Autodesk Inventor part; units mm, degrees
ref_plane "YZ Plane" through (0, 0, 0) normal (1, 0, 0) x (0, 1, 0)
ref_plane "XZ Plane" through (0, 0, 0) normal (0, 1, 0) x (-1, 0, 0)
ref_plane "XY Plane" through (0, 0, 0) normal (0, 0, 1) x (1, 0, 0)
sketch "Sketch1" plane through (0, 0, 0) normal (0, 1, 0) x (-1, 0, 0)
  line L0 (217.0075, 238.5115) -> (-11.2469, 238.5115)
  line L1 (-36.6469, 213.1115) -> (-36.6469, 88.1828)
  line L2 (-11.5925, 62.7851) -> (215.7472, 62.7851)
  line L3 (241.1469, 88.0591) -> (241.1469, 213.1428)
  arc A0 (217.0075, 238.5115) -> (241.1469, 213.1428) centre (242.4075, 238.5115) ccw
  arc A1 (241.1469, 88.0591) -> (215.7472, 62.7851) centre (241.1469, 62.6591) ccw
  arc A2 (-36.6469, 213.1115) -> (-11.2469, 238.5115) centre (-36.6469, 238.5115) ccw
  arc A3 (-11.5925, 62.7851) -> (-36.6469, 88.1828) centre (-36.9925, 62.7851) ccw
  circle A4 centre (215.7469, 150.6529) radius 9.525
  circle A5 centre (215.7469, 150.6529) radius 6.35
  point P0 (0, 0)
  dimension "d6" = 227.3398
  dimension "d7" = 277.7939
  dimension "d10" = 125.0838
  dimension "d11" = 175.7264
  dimension "d12" = 19.05
  dimension "d13" = 12.7
  dimension "d14" = 87.8586
  dimension "d15" = 25.4
extrude "Extrusion1" add sketch "Sketch1" along normal blind 25.4 contours A0 L3 A1 L2 A3 L1 A2 L0 | A4 | A5
extrude "Extrusion2" cut sketch "Sketch1" along normal blind 5.08 contours A5
sketch "Sketch2" plane through (0, 0, 0) normal (0, -1, 0) x (1, 0, 0)
  point P0 (0, 0)
sketch "Sketch3" plane through (0, 0, 0) normal (0, -1, 0) x (1, 0, 0)
  line L0 (-39.8772, 113.6871) -> (5.2014, 113.6871)
  line L1 (5.2014, 113.6871) -> (5.2014, 191.46)
  line L2 (5.2014, 191.46) -> (-39.8772, 191.46)
  line L3 (-39.8772, 191.46) -> (-39.8772, 113.6871)
  point P0 (0, 0)
extrude "Extrusion3" add sketch "Sketch3" along normal blind 177.8
sketch "Sketch4" plane through (-39.8772, 0, 191.46) normal (0, 0, 1) x (1, 0, 0)
  point P0 (39.8772, 0)
sketch "Sketch5" plane through (-39.8772, 0, 191.46) normal (0, 0, 1) x (1, 0, 0)
  circle A0 centre (24.2438, -148.3134) radius 6.35
  point P0 (39.8772, 0)
  dimension "d20" = 12.7
hole "Hole1" at (-15.6334, -148.3134, 191.46) direction (0, 0, -1) diameter 12.7 end through all counterbore diameter 19.05 counterbore depth 3.048
shell "Shell1" thickness 2.54 removed faces 2 at (-24.851, -177.8, 139.6114) at (-15.1224, -154.6429, 163.5037)
sketch "Sketch6" plane through (-39.8772, 0, 191.46) normal (0, 0, 1) x (1, 0, 0)
  circle A0 centre (24.2438, -27.5812) radius 6.35
  point P0 (39.8772, 0)
  dimension "d29" = 12.7
hole "Hole2" at (-15.6334, -27.5812, 191.46) direction (0, 0, -1) diameter 12.7 end through all counterbore diameter 19.05 counterbore depth 3.048
shell "Shell2" thickness 2.54 removed faces 3 at (-143.2625, 25.4, 176.3813) at (-140.9901, 22.86, 175.1392) at (-153.6846, 2.54, 191.1872)
properties part number "BASE"
Design review of the part built by this model. Coordinates are the model's own, in mm. A direction names the side the tool comes from. Coordinates: 2 decimals unless noted, no trailing zeros. Loops run counter-clockwise (first coordinate to the right, second up) from the corner with the lowest first, then second, coordinate; pieces in that order, holes last.
Item 1: Wall thickness on L1, parallel to Z at x = -23, y = -119; L2, parallel to X at y = -81, z = 184; L3, parallel to X at y = 10, z = 97.5: over which ranges is each line inside the solid? List them lowest first.
Completed:
L1: z = 113.69 to 116.23, 188.92 to 191.46
L2: x = -39.88 to -37.34, 2.66 to 5.2
L3: x = -241.15 to -238.61, 34.11 to 36.65
Item 2: Draft analysis for pull direction X (two halves, no side actions). For faces 5 (the cylindrical face through (18.49, 12.52, 220.75)), 6 (the cylindrical face through (-19.26, -159.82, 187.37)), 7 (the flat face through (-100, 13, 62.785)), 8 (the flat face through (-241.147, 13, 150)), state which applies: pulls with the +X half, pulls with the -X half, needs draft (parallel to the pull), parting line crosses it, or undercut.
Completed:
face 5: pulls with the +X half
face 6: undercut
face 7: needs draft
face 8: pulls with the -X half
Item 3: Add section D-D (z = 94.5). Write out the cut boundary in (x, y), and give its area (3 significant figures).
Completed:
outline: (-241.15, 0) - (36.65, 0) - (36.65, 25.4) - (34.11, 25.4) - (34.11, 2.54) - (-238.61, 2.54) - (-238.61, 25.4) - (-241.15, 25.4) - close
area: 822 mm2
Item 4: Add section B-B (z = 125). Write out the cut boundary in (x, y), and give its area (3 significant figures).
Completed:
outline: (-241.15, 0) - (-39.88, 0) - (-39.88, -177.8) - (-37.34, -177.8) - (-37.34, 2.54) - (-238.61, 2.54) - (-238.61, 25.4) - (-241.15, 25.4) - close; (2.66, -177.8) - (5.2, -177.8) - (5.2, 0) - (36.65, 0) - (36.65, 25.4) - (34.11, 25.4) - (34.11, 2.54) - (2.66, 2.54) - close
area: 1,620 mm2
Item 5: Add section C-C (x = -197.5). Write out the cut boundary in (y, z), and give its area (3 significant figures).
Completed:
outline: (0, 62.79) - (25.4, 62.79) - (25.4, 65.33) - (2.54, 65.33) - (2.54, 235.97) - (25.4, 235.97) - (25.4, 238.51) - (0, 238.51) - close
area: 562 mm2
Item 6: Clearance check with flat-ended pins moving along their axes: pin 1 (11.5 mm diameter, centred on x = -215.75, z = 150.65, fed in from +Y); pin 2 (14.5 mm diameter, centred on x = -15.63, y = -148.31, fed in from +Z); pin 3 (16.5 mm diameter, centred on x = -15.63, y = -27.58, fed in from -Z). State where each tip first meets the part, or that it passes through.
Completed:
pin 1: stops at y = 7.62
pin 2: stops at z = 188.41
pin 3: stops at z = 113.69
Item 7: For faces 1 (the flat face through (5.201, -88, 152)), 2 (the flat face through (-104, 14, 235.972)), 3 (the flat face through (-216, 5.08, 151)), 4 (the flat face through (-10, -154, 185.872)), list the 3-axis set-ups (+Z, -Z, +X, -X, +Y, -Y) from which the entire face can be reached by the end or side of a thin tool; tool diameter is ignored.
Completed:
face 1: +Z, -Z, +X, -Y
face 2: +Y
face 3: -Y
face 4: +Y, -Y
Item 8: Add section A-A (y = -107). Write out the cut boundary in (x, z), and give its area (3 significant figures).
Completed:
outline: (-39.88, 113.69) - (5.2, 113.69) - (5.2, 191.46) - (-39.88, 191.46) - close; hole (-37.34, 116.23) - (2.66, 116.23) - (2.66, 188.92) - (-37.34, 188.92) - close
area: 598 mm2
